from build123d import *

# Parameters (mm, degrees)
SKETCH2_W           = 10
SKETCH2_H           = 45
SKETCH2_R           = 1.75
BOSS_EXTRUDE1_DEPTH = 3
SKETCH3_W           = 10
SKETCH3_H           = 20
BOSS_EXTRUDE2_DEPTH = 25
SKETCH4_R           = 6
CUT_EXTRUDE1_DEPTH  = 10
SKETCH5_R           = 1
CUT_EXTRUDE2_DEPTH  = 20


with BuildPart() as part:
    # Sketch2 → Boss-Extrude1 (new body)
    with BuildSketch(Plane(origin=(0, 0, 0), x_dir=(1, 0, 0), z_dir=(0, 1, 0))):
        Rectangle(SKETCH2_W, SKETCH2_H)
        with Locations(Location((0, 17.5, 0), (0, 0, 270))):
            Circle(SKETCH2_R, mode=Mode.SUBTRACT)
        with Locations(Location((0, -17.5, 0), (0, 0, 270))):
            Circle(SKETCH2_R, mode=Mode.SUBTRACT)
    extrude(amount=BOSS_EXTRUDE1_DEPTH)

    # Sketch3 → Boss-Extrude2 (add)
    with BuildSketch(Plane(origin=(0, 3, 0), x_dir=(1, 0, 0), z_dir=(0, 1, 0))):
        Rectangle(SKETCH3_W, SKETCH3_H)
    extrude(amount=BOSS_EXTRUDE2_DEPTH)

    # Sketch4 → Cut-Extrude1 (cut)
    with BuildSketch(Plane.ZY.offset(5)):
        with Locations((0, 18)):
            Circle(SKETCH4_R)
    extrude(amount=-CUT_EXTRUDE1_DEPTH, mode=Mode.SUBTRACT)

    # Sketch5 → Cut-Extrude2 (cut)
    with BuildSketch(Plane.XY.offset(10)):
        with Locations((0, 18)):
            Circle(SKETCH5_R)
    extrude(amount=-CUT_EXTRUDE2_DEPTH, mode=Mode.SUBTRACT)


solid = part.part
Can you work these out from the model? Positions are in its coordinate system, mm. A direction names the side the tool comes from. Give positions to 0.01 mm unless a question says otherwise; leave off trailing zeros. Order: outer loops, then holes, each group sorted by start corner. A loop starts at its lowest first (then second) coordinate and runs counter-clockwise, first axis right, second up. Notation, with made-up numbers: M 35.5,58 L 44.5,58 A16 cw 44.5,75 Z; hole C -19.75,65.25 d6. An arc over 180 degrees is marked long. One line per question, with ' | ' between items.
Item 1: We'd pull the mould along Y, two halves only. Please class faces 4 (the face through (-0.07, 19.802, 5.723)), 5 (the face through (0, 0, 0)), 6 (the face through (0, 1, -22.5)), 7 (the face through (0, 28, 0)): released by +Y, released by -Y, zero draft, split by the parting line, or undercut.
Answer block:
face 4: undercut | face 5: released by -Y | face 6: zero draft | face 7: released by +Y
Item 2: Suppose I cut it at C-C, the plane x = -2.25. Write out the boundary of the cut face in (y, z).
Answer block:
outline: M 0,-22.5 L 3,-22.5 L 3,-10 L 28,-10 L 28,10 L 3,10 L 3,22.5 L 0,22.5 Z; hole C 18,0 d12
Item 3: Suppose I cut it at D-D, the plane z = -17.5. Write out the boundary of the cut face in (x, y), then the cut area to 3 significant figures.
Answer block:
outline: M -5,0 L -1.75,0 L -1.75,3 L -5,3 Z; M 1.75,0 L 5,0 L 5,3 L 1.75,3 Z | area: 19.5 mm2
Item 4: Please list where these lines run through material, in increasing order: L1, parallel to X at y = 2.05, z = 17.5; L2, parallel to X at y = 18, z = -8.5; L3, parallel to Y at x = 0, z = -8.8.
Answer block:
L1: x = -5 to -1.75, 1.75 to 5 | L2: x = -5 to -1, 1 to 5 | L3: y = 0 to 17, 19 to 28
Item 5: Suppose I cut it at A-A, the plane x = 0. Write out the boundary of the cut face in (y, z), then the cut area to 3 significant figures.
Answer block:
outline: M 0,-22.5 L 3,-22.5 L 3,-19.25 L 0,-19.25 Z; M 0,-15.75 L 3,-15.75 L 3,-10 L 17,-10 L 17,-5.92 A6 cw 17,5.92 L 17,10 L 3,10 L 3,15.75 L 0,15.75 Z; M 0,19.25 L 3,19.25 L 3,22.5 L 0,22.5 Z; M 19,-10 L 28,-10 L 28,10 L 19,10 L 19,5.92 A6 cw 19,-5.92 Z | area: 485 mm2
Item 6: Suppose I cut it at B-B, the plane y = 18. Write out the boundary of the cut face in (x, z), then the cut area to 3 significant figures.
Answer block:
outline: M -5,-10 L -1,-10 L -1,-6 L -5,-6 Z; M -5,6 L -1,6 L -1,10 L -5,10 Z; M 1,-10 L 5,-10 L 5,-6 L 1,-6 Z; M 1,6 L 5,6 L 5,10 L 1,10 Z | area: 64.0 mm2
Item 7: For faces 1 (the face through (0, 15, -10)), 2 (the face through (5, 11, 0)), 3 (the face through (0, 3, 15)), which set-ups out of +Z, -Z, +X, -X, +Y, -Y let a thin tool reach every point of the face, with its end or its side?
Answer block:
face 1: -Z, +X, -X, +Y | face 2: +Z, -Z, +X, +Y, -Y | face 3: +Z, +X, -X, +Y
Item 8: I'm going to push flat-ended pins straight in: pin 1 Ø2.5 at (x, y) = (0, 18) entering from +Z; pin 2 Ø3 at (x, z) = (0, 17.5) entering from +Y; pin 3 Ø3 at (x, y) = (0, 18) entering from -Z. Where does each tip first touch, or does it pass through?
Answer block:
pin 1: stops at z = 10 | pin 2: passes through | pin 3: stops at z = -10
